Autodesk Inventor part; units mm, degrees
ref_plane "YZ Plane" through (0, 0, 0) normal (1, 0, 0) x (0, 1, 0)
ref_plane "XZ Plane" through (0, 0, 0) normal (0, 1, 0) x (-1, 0, 0)
ref_plane "XY Plane" through (0, 0, 0) normal (0, 0, 1) x (1, 0, 0)
sketch "Sketch1" plane through (0, 0, 0) normal (0, 1, 0) x (-1, 0, 0)
  line L0 (0, 0) -> (9.899, 0)
  line L1 (9.899, 0) -> (9.899, -17.899)
  line L2 (9.899, -17.899) -> (0, -17.899)
  line L3 (0, -17.899) -> (0, 0)
  line L4 (0.5, -0.5) -> (9.399, -0.5)
  line L5 (9.399, -0.5) -> (9.399, -17.399)
  line L6 (9.399, -17.399) -> (0.5, -17.399)
  line L7 (0.5, -17.399) -> (0.5, -0.5)
  dimension "d0" = 9.899
  dimension "d1" = 17.899
  dimension "d2" = 16.899
  dimension "d3" = 8.899
  dimension "d4" = 0.5
  dimension "d5" = 0.5
sketch "Sketch3" plane through (0, 0, 0) normal (1, 0, 0) x (0, 1, 0)
  arc A0 (0, 0) -> (13, 13) centre (0, 13) ccw
  line L0 (0, 13) -> (13, 13) construction
  line L1 (0, 13) -> (0, 0) construction
  dimension "d6" = 90
  dimension "d7" = 13
sweep "Sweep1" add profiles "Sketch1" path "Sketch3"
extrude "Extrusion1" add sketch "Sketch1" against normal blind 16.55
ref_plane "Work Plane1" through (-9.899, 13, 13) normal (0, 0, 1) x (1, 0, 0)
sketch "Sketch4" plane through (-9.899, 13, 13) normal (0, 0, 1) x (1, 0, 0)
  line L0 (0, 0) -> (9.899, 0)
  line L1 (0, 0) -> (0, 17.899)
  line L2 (0, 17.899) -> (9.899, 17.899)
  line L3 (9.899, 17.899) -> (9.899, 0)
  line L4 (0.5, 17.399) -> (9.399, 17.399)
  line L5 (9.399, 17.399) -> (9.399, 0.5)
  line L6 (9.399, 0.5) -> (0.5, 0.5)
  line L7 (9.399, 0.5) -> (0.5, 0.5)
  line L8 (0.5, 0.5) -> (0.5, 17.399)
extrude "Extrusion2" add sketch "Sketch4" along normal blind 16.55
properties part number "curved waveguide"
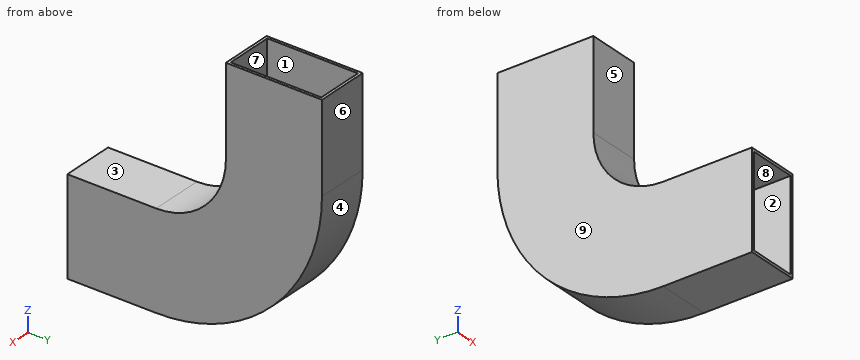
Read the model definition and answer for the solid it produces. Units are mm, in the model's axes. Face numbers are marked on the shaded views. A direction names the side the tool comes from. Give positions to 0.01 mm unless a question says otherwise; leave off trailing zeros. Write each loop counter-clockwise with the first axis right and the second up, starting at its lowest first coordinate (ties: lowest second). Pieces come first, ordered by that corner, then holes. Notation, with made-up numbers: M 4,-7.75 L 17,-7.75 A24 ccw 17,16.25 Z; hole C -13,55.5 d6. An arc over 180 degrees is marked long. One line per item, written item: value. Start each with the question number.
(1) Find the intervals of material crossed by line 1 (X direction, y = 19, z = -10); line 2 (Y direction, x = -4.75, z = 16.5); line 3 (Z direction, x = -1.5, y = -11.5), in increasing order.
(2) Determine the mould class of the marked faces 1, 2, 3 and 4 for opening direction Y: pulls with the +Y half, pulls with the -Y half, needs draft (parallel to the pull), parting line crosses it, or undercut.
(3) Find section C-C (z = 19). Determine the outline of the cut face in (x, y), plus the area to 3 significant figures.
(4) A tool of negligible diameter and unlimited length cuts with its end or side. For the marked faces 5, 6, 7, 8 and 9, from which of +Z, -Z, +X, -X, +Y, -Y can it reach the whole face along a straight path? Write none if from no direction.
(5) Flat-ended cylindrical pins translate along their axes: pin 1 Ø3 at (x, y) = (-3, 7.5) entering from -Z; pin 2 Ø5 at (x, y) = (-5, 23.5) entering from +Z; pin 3 Ø1.5 at (x, z) = (-3.5, -7.5) entering from +Y. Find the tip coordinate at first contact, or state that the pin passes through.
(6) Find section A-A (x = -6.75). Determine the outline of the cut face in (y, z).
(7) Find section B-B (y = -11). Determine the outline of the cut face in (x, z).
(8) Find section D-D (y = 22). Determine the outline of the cut face in (x, z).
Results below:
1. line 1: x = -9.9 to -9.4, -0.5 to 0
1. line 2: y = 13 to 13.5, 30.4 to 30.9
1. line 3: z = -17.9 to -17.4, -0.5 to 0
2. face 1: undercut
2. face 2: undercut
2. face 3: needs draft
2. face 4: pulls with the +Y half
3. outline: M -9.9,13 L 0,13 L 0,30.9 L -9.9,30.9 Z; hole M -9.4,13.5 L -0.5,13.5 L -0.5,30.4 L -9.4,30.4 Z
3. area: 26.8 mm^2
4. face 5: +Z, +X, -X, -Y
4. face 6: +Z, -Z, +X, -X, +Y
4. face 7: +Z
4. face 8: -Y
4. face 9: +Z, -Z, -X, +Y, -Y
5. pin 1: stops at z = -17.31
5. pin 2: stops at z = -2.75
5. pin 3: stops at y = 23.76
6. outline: M -16.55,-17.9 L 0,-17.9 A30.9 ccw 30.9,13 L 30.9,29.55 L 30.4,29.55 L 30.4,13 A30.4 cw 0,-17.4 L -16.55,-17.4 Z; M -16.55,-0.5 L 0,-0.5 A13.5 ccw 13.5,13 L 13.5,29.55 L 13,29.55 L 13,13 A13 cw 0,0 L -16.55,0 Z
7. outline: M -9.9,-17.9 L 0,-17.9 L 0,0 L -9.9,0 Z; hole M -9.4,-17.4 L -0.5,-17.4 L -0.5,-0.5 L -9.4,-0.5 Z
8. outline: M -9.9,-8.7 L 0,-8.7 L 0,29.55 L -0.5,29.55 L -0.5,-7.98 L -9.4,-7.98 L -9.4,29.55 L -9.9,29.55 Z
